Can you work these out from the drawing? Everything is in mm from the part's minimum corner. Round coordinates to 2 decimals unless told otherwise and drop trailing zeros. Loops run counter-clockwise (first coordinate to the right, second up) from the corner with the lowest first, then second, coordinate; pieces in that order, holes last. Notation, with made-up numbers: (-17.75, 16.5) -> (-11.75, 16.5) arc R12 cw to (-11.75, 37.5) -> close; hole circle Ø8 at (42, 48). An arc over 180 degrees is marked (long way). One line per item, written item: value.
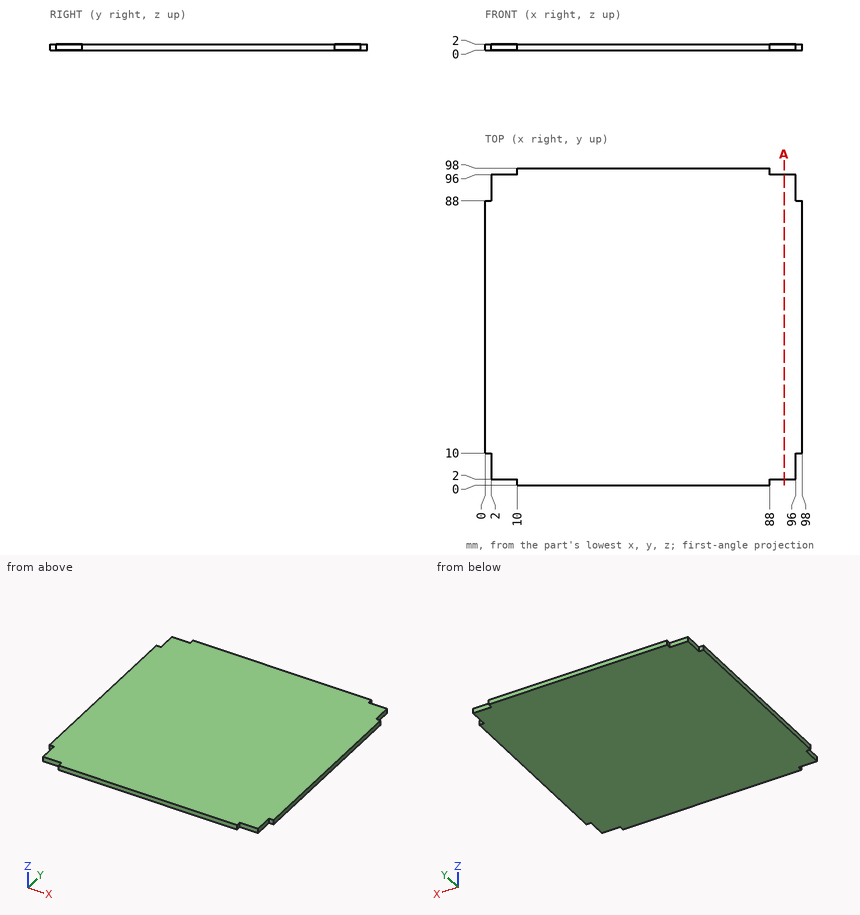
(1) Please list where this line runs through material, in increasing order: L1, parallel to Y at x = 90, z = 0.6.
Results below:
L1: y = 2 to 96
(2) For pin 1 Ø0.6 at (y, z) = (91, 0.5) entering from +X; pin 2 Ø0.6 at (x, z) = (97, 0.5) entering from -Y; pin 3 Ø0.6 at (y, z) = (1.5, 0.5) entering from +X, each with a flat end and sliding along its axis, tell me the tip position at first contact or that it passes through.
Results below:
pin 1: stops at x = 96
pin 2: stops at y = 10
pin 3: stops at x = 88
(3) Imagine slicing it at A-A on x = 92.5. Write out the boundary of the cut face in (y, z), then the cut area to 3 significant figures.
Results below:
outline: (2, 0) -> (96, 0) -> (96, 2) -> (2, 2) -> close
area: 188 mm²
